Read the model definition and answer for the solid it produces. Units are mm, in the model's axes. Coordinates: 2 decimals unless noted, no trailing zeros. Write each loop counter-clockwise with the first axis right and the second up, starting at its lowest first coordinate (ties: lowest second). Pieces come first, ordered by that corner, then holes.
Item 1: Section A-A (z = -242) is taken. Give the vertices of the cut face in (x, y).
Item 2: Section B-B (x = -6.5) is taken. Give the vertices of the cut face in (y, z), then the cut area to 4 significant figures.
Item 3: Each of these flat-tipped pins is pushed along its axis until it touches: P1, Ø23, axis at y = 0, z = 275, coming from the +X side; P2, Ø24, axis at x = -3.5, y = 11.5, coming from the +Z side; P3, Ø6, axis at y = 18, z = -93, coming from the -X side. Where does it stop, or does it pass through?
Item 4: Straight lines are drawn through the part: probe 1 along Z at (x, y) = (19, 0); probe 2 along Y at (x, z) = (-20.25, 275); probe 3 along X at (y, z) = (10, -311). For each, find the intervals that lie inside material, in ascending order.
from build123d import *

# Parameters (mm, degrees)
SKETCH1_R           = 10
BOSS_EXTRUDE1_DEPTH = 24
SKETCH2_W           = 25
SKETCH2_H           = 60
SKETCH2_W_2         = 30
CUT_EXTRUDE1_DEPTH  = 429.603546416
SKETCH3_R           = 15
BOSS_EXTRUDE2_DEPTH = 37.5


with BuildPart() as part:
    # Sketch1 → Boss-Extrude1 (new, symmetric)
    with BuildSketch(Plane(origin=(0, 0, 0), x_dir=(0, 0, -1), z_dir=(1, 0, 0))):
        with BuildLine():
            Line((-275, 25), (400, 25))
            ThreePointArc((400, 25), (425, 0), (400, -25))
            Line((400, -25), (-275, -25))
            ThreePointArc((-275, -25), (-300, 0), (-275, 25))
        make_face()
        with Locations((-275, 0)):
            Circle(SKETCH1_R, mode=Mode.SUBTRACT)
        with Locations((400, 0)):
            Circle(SKETCH1_R, mode=Mode.SUBTRACT)
    extrude(amount=BOSS_EXTRUDE1_DEPTH, both=True)

    # Sketch2 → Cut-Extrude1 (cut, through all)
    with BuildSketch(Plane(origin=(0, 25, 0), x_dir=(1, 0, 0), z_dir=(0, 1, 0))):
        with Locations((0, 395)):
            Rectangle(SKETCH2_W, SKETCH2_H)
        with Locations((0, -270)):
            Rectangle(SKETCH2_W_2, SKETCH2_H)
    extrude(amount=-CUT_EXTRUDE1_DEPTH, mode=Mode.SUBTRACT)

    # Sketch3 → Boss-Extrude2 (add, symmetric)
    with BuildSketch(Plane(origin=(0, 0, 0), x_dir=(0, 0, -1), z_dir=(1, 0, 0))):
        Circle(SKETCH3_R)
    extrude(amount=BOSS_EXTRUDE2_DEPTH, both=True)


solid = part.part
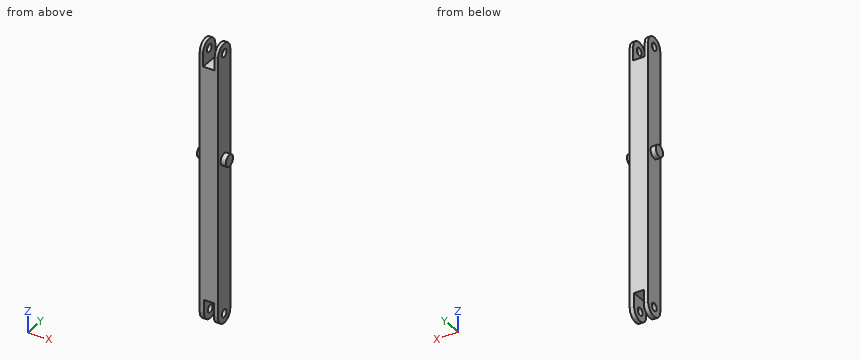
Established:
1. outline: (-24, -25) - (24, -25) - (24, 25) - (-24, 25) - close
2. outline: (-25, -365) - (25, -365) - (25, 240) - (-25, 240) - close
2. area: 30,250 mm2
3. P1: stops at x = 24
3. P2: stops at z = 298.66
3. P3: stops at x = -24
4. probe 1: z = -425 to -410, -390 to 265, 285 to 300
4. probe 2: y = -25 to -10, 10 to 25
4. probe 3: x = -24 to 24
